The drawing under review shows one solid part. Ordinate dimensions are in mm from its lowest x, y, z. A direction names the side the tool comes from. Give positions to 0.01 mm unless a question says otherwise; leave off trailing zeros. Write each loop counter-clockwise with the first axis right and the second up, starting at its lowest first coordinate (ties: lowest second). Pieces come first, ordered by that corner, then holes.
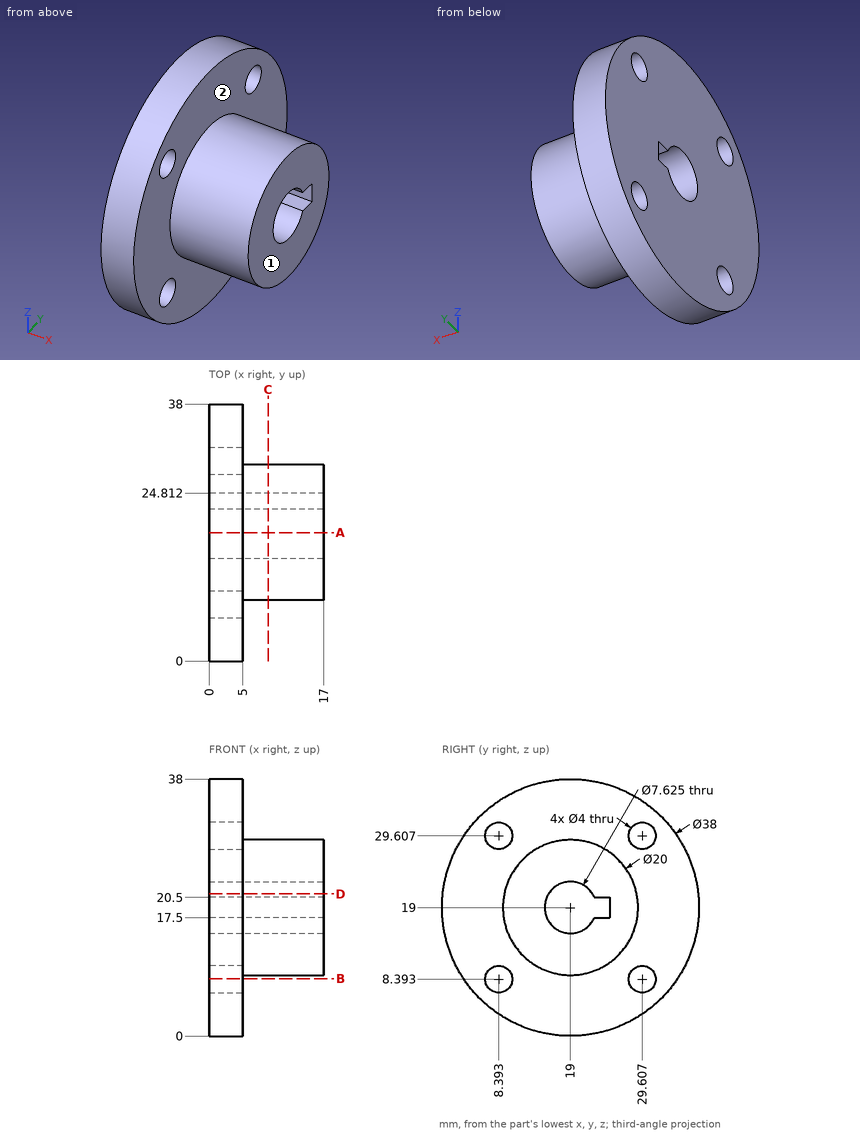
1) Tool access review of the marked faces 1 and 2: name each direction out of +Z, -Z, +X, -X, +Y, -Y from which nothing blocks a thin tool from reaching the whole face with its end or side.
2) Consider section B-B, the plane z = 8.5. Give the boundary of the cut face in (x, y) (1 decimal).
3) Insertion check: pin 1 (3 mm diameter, centred on x = 14.5, z = 11, fed in from +Y); pin 2 (5 mm diameter, centred on y = 8.39, z = 8.39, fed in from -X); pin 3 (1.2 mm diameter, centred on x = 9.5, y = 24, fed in from -Z); pin 4 (6.5 mm diameter, centred on y = 29.61, z = 8.39, fed in from +X). Each pin has a flat end and moves straight along its axis. Give the tip position at first contact, or say it passes through.
4) Consider section D-D, the plane z = 21. Give the boundary of the cut face in (x, y) (1 decimal).
5) Consider section A-A, the plane y = 19. Give the boundary of the cut face in (x, z).
6) To check wall thickness, follow probe 1 along Y at (x, z) = (5.75, 19); probe 2 along Y at (x, z) = (1.75, 7); probe 3 along Z at (x, y) = (4, 30) (1 decimal). State the ranges of each line that lie inside material, in increasing order.
7) Consider section C-C, the plane x = 8.75. Give the boundary of the cut face in (y, z) (1 decimal).
Answer block:
1. face 1: +Z, -Z, +X, +Y, -Y
1. face 2: +X
2. outline: (0, 3.2) - (5, 3.2) - (5, 6.4) - (0, 6.4) - close; (0, 10.4) - (5, 10.4) - (5, 27.6) - (0, 27.6) - close; (0, 31.6) - (5, 31.6) - (5, 34.8) - (0, 34.8) - close
3. pin 1: stops at y = 26.6
3. pin 2: stops at x = 0
3. pin 3: stops at z = 10.02
3. pin 4: stops at x = 5
4. outline: (0, 0.1) - (5, 0.1) - (5, 9.2) - (17, 9.2) - (17, 15.8) - (0, 15.8) - close; (0, 22.2) - (17, 22.2) - (17, 28.8) - (5, 28.8) - (5, 37.9) - (0, 37.9) - close
5. outline: (0, 0) - (5, 0) - (5, 9) - (17, 9) - (17, 15.19) - (0, 15.19) - close; (0, 22.81) - (17, 22.81) - (17, 29) - (5, 29) - (5, 38) - (0, 38) - close
6. probe 1: y = 9 to 15.19, 24.81 to 29
6. probe 2: y = 4.27 to 6.96, 9.83 to 28.17, 31.04 to 33.73
6. probe 3: z = 3.5 to 6.4, 10.4 to 27.6, 31.6 to 34.5
7. outline: circle Ø20 at (19, 19); hole (22.5, 17.5) - (24.8, 17.5) - (24.8, 20.5) - (22.5, 20.5) arc R3.8 ccw (long way) to start
